Geometry check sheet. Reference: drawing and pictorial views, mm from the part's lowest x, y, z. A direction names the side the tool comes from. Coordinates: 2 decimals unless noted, no trailing zeros. Loops run counter-clockwise (first coordinate to the right, second up) from the corner with the lowest first, then second, coordinate; pieces in that order, holes last. Notation, with made-up numbers: (68.25, 69) - (113.25, 69) arc R13 ccw to (113.25, 91) - close; hole circle Ø10 at (47.25, -39). An arc over 180 degrees is marked (long way). One line per item, written item: value.
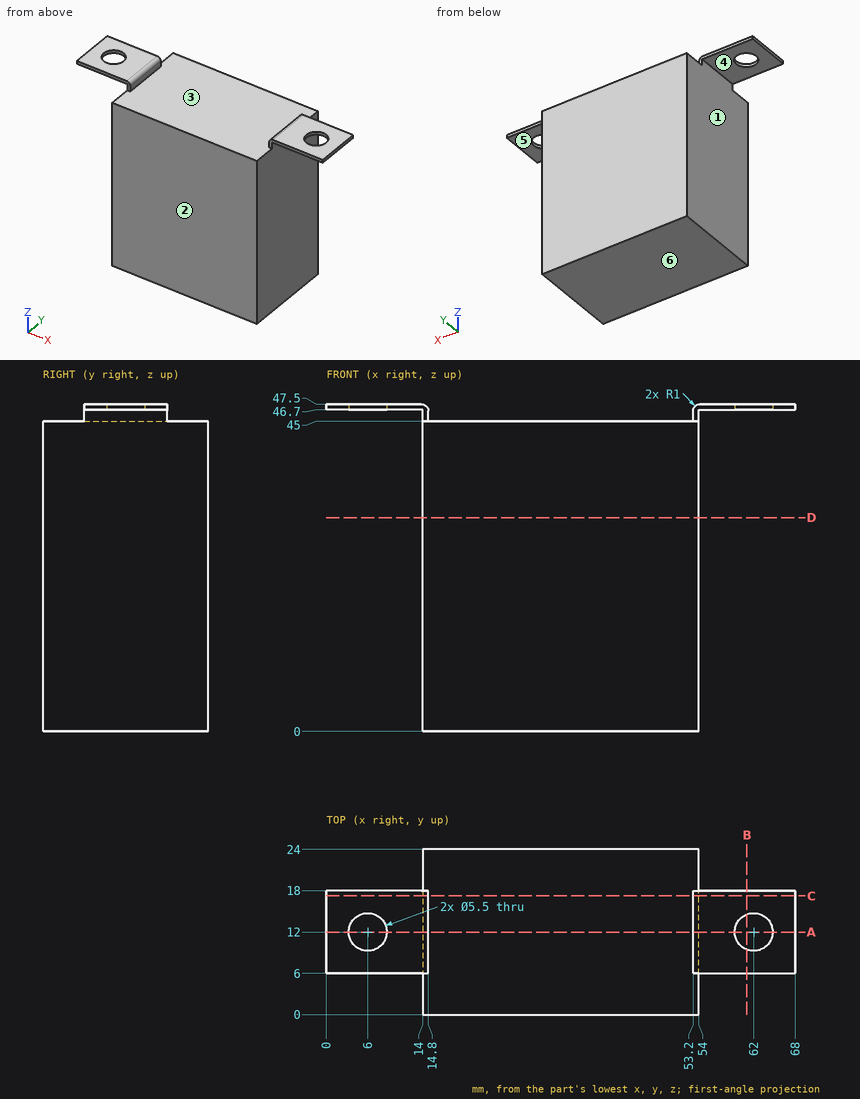
(1) Go/stop test with flat-tipped pins: pin 1 Ø6 at (y, z) = (16, 37.5) entering from +X; pin 2 Ø2 at (x, z) = (59.5, 46.5) entering from -Y; pin 3 Ø9.5 at (x, y) = (4.5, 10) entering from -Z; pin 4 Ø3.5 at (x, y) = (6, 12) entering from +Z. Record where each tip stops, or that it passes through.
Reply:
pin 1: x = 54
pin 2: y = 6
pin 3: z = 46.7
pin 4: through
(2) Cross-section at D-D on z = 31. Record the cut outline in (x, y).
Reply:
outline: (14, 0) - (54, 0) - (54, 24) - (14, 24) - close
(3) Cross-section at C-C on y = 17.25. Record the cut outline in (x, z).
Reply:
outline: (0, 46.7) - (14, 46.7) - (14, 0) - (54, 0) - (54, 46.7) - (68, 46.7) - (68, 47.5) - (54.2, 47.5) arc R1 ccw to (53.2, 46.5) - (53.2, 45) - (14.8, 45) - (14.8, 46.5) arc R1 ccw to (13.8, 47.5) - (0, 47.5) - close
(4) Material ranges on probe 1 along Y at (x, z) = (6, 47); probe 2 along X at (y, z) = (12, 47.05); probe 3 along X at (y, z) = (4.75, 4), recorded low to high. Write a range as from..to.
Reply:
probe 1: 6..9.25, 14.75..18
probe 2: 0..3.25, 8.75..14.64, 53.36..59.25, 64.75..68
probe 3: 14..54
(5) Cross-section at A-A on y = 12. Record the cut outline in (x, z), and give its area (3 significant figures).
Reply:
outline: (0, 46.7) - (3.25, 46.7) - (3.25, 47.5) - (0, 47.5) - close; (8.75, 46.7) - (14, 46.7) - (14, 0) - (54, 0) - (54, 46.7) - (59.25, 46.7) - (59.25, 47.5) - (54.2, 47.5) arc R1 ccw to (53.2, 46.5) - (53.2, 45) - (14.8, 45) - (14.8, 46.5) arc R1 ccw to (13.8, 47.5) - (8.75, 47.5) - close; (64.75, 46.7) - (68, 46.7) - (68, 47.5) - (64.75, 47.5) - close
area: 1,820 mm2
(6) Access from +Z, -Z, +X, -X, +Y, -Y to the whole of each face (thin tool, end or side, straight path). Record for the marked faces 4, 5 and 6.
Reply:
face 4: -Z, -X, +Y, -Y
face 5: -Z, +X, +Y, -Y
face 6: -Z, +X, -X, +Y, -Y
(7) Release check for a two-part mould opening along X. For the marked faces 1, 2 and 3 record: pulls with the +X half, pulls with the -X half, needs draft (parallel to the pull), parting line crosses it, or undercut.
Reply:
face 1: pulls with the -X half
face 2: needs draft
face 3: undercut
(8) Cross-section at B-B on x = 61. Record the cut outline in (y, z), and give its area (3 significant figures).
Reply:
outline: (6, 46.7) - (9.44, 46.7) - (9.44, 47.5) - (6, 47.5) - close; (14.56, 46.7) - (18, 46.7) - (18, 47.5) - (14.56, 47.5) - close
area: 5.50 mm2
